Input: part model. Units: mm. Frame: model coordinates. A direction names the side the tool comes from. Give positions to 0.01 mm unless a question says otherwise; leave off trailing zeros. Write each loop counter-clockwise with the first axis right and the second up, starting at its lowest first coordinate (ties: lowest second). Pieces come first, ordered by that corner, then holes. Notation, with made-up numbers: (-38.75, 70) - (17.25, 70) arc R33 ccw to (17.25, 106) - close; hole circle Ø10 at (3, 30.25). An arc over 180 degrees is marked (long way). Use a Markdown table: item, result. Add a question column.
1. Material intervals for probe 1 along X at (y, z) = (3.6, -5); probe 2 along X at (y, z) = (1.4, 25.5); probe 3 along Z at (x, y) = (6, 1.45), sorted ascending.
2. Section query A-A, the plane z = 6.5. Return loops of the section in (x, y).
3. Mould query, pull axis X, two halves, no side actions, for faces 1 (the flat face through (13.804, 1.972, 24.362)), 2 (the flat face through (-28, 2, 0)), 3 (the flat face through (-13, 4, 24)), 4 (the flat face through (-13.21, 1.97, -23.32)). Classes: released by +X, released by -X, zero draft, split by the parting line, or undercut.
4. Set-up query: faces 5 (the flat face through (26.8, 2, 0)), 6 (the flat face through (-13.804, 1.972, -24.362)). Return all of +Z, -Z, +X, -X, +Y, -Y with unobstructed straight access to the full face (end or side cutting, diameter ignored); none if empty.
5. Section query B-B, the plane x = -2.5. Return loops of the section in (y, z), plus the area to 3 significant figures.
6. Pin query (flat end, axial travel): pin 1 (1.5 mm diameter, centred on x = 17.5, y = 2.5, fed in from +Z). Return the tip coordinate at first contact, or that it passes through.
```python
from build123d import *

# Parameters (mm, degrees)
RESSALTO_EXTRUS_O1_DEPTH = 4
ESBO_O2_R                = 1
CORTE_EXTRUS_O1_DEPTH    = 71.578561429


with BuildPart() as part:
    # Esboço1 → Ressalto-extrusão1 (new body)
    with BuildSketch(Plane(origin=(0, 0, 0), x_dir=(1, 0, 0), z_dir=(0, 1, 0))):
        Polygon((28, -16.165807537), (28, 16.165807537), (0, 32.331615075), (-28, 16.165807537), (-28, -16.165807537), (0, -32.331615075), align=None)
        Polygon((26.8, 15.472987214), (0, 30.945974429), (-26.8, 15.472987214), (-26.8, -15.472987214), (0, -30.945974429), (26.8, -15.472987214), align=None, mode=Mode.SUBTRACT)
    extrude(amount=RESSALTO_EXTRUS_O1_DEPTH)

    # Esboço2 → Corte-extrusão1 (cut, through all)
    with BuildSketch(Plane(origin=(-14, 0, 24.248711306), x_dir=(0.8660254037844387, 0, 0.49999999999999994), z_dir=(-0.4999999999999999, 0, 0.8660254037844386))):
        with Locations((0, 2)):
            Circle(ESBO_O2_R)
    extrude(amount=-CORTE_EXTRUS_O1_DEPTH, mode=Mode.SUBTRACT)


solid = part.part
```
Result sheet:
| question | item | result |
|---|---|---|
| 1 | probe 1 | x = -28 to -26.8, 26.8 to 28 |
| 1 | probe 2 | x = -11.83 to -9.43, 9.43 to 11.83 |
| 1 | probe 3 | z = -28.87 to -27.48, 27.48 to 28.87 |
| 2 | outline | (-28, 0) - (-26.8, 0) - (-26.8, 4) - (-28, 4) - close; (26.8, 0) - (28, 0) - (28, 4) - (26.8, 4) - close |
| 3 | face 1 | released by +X |
| 3 | face 2 | released by -X |
| 3 | face 3 | zero draft |
| 3 | face 4 | undercut |
| 4 | face 5 | +Y, -Y |
| 4 | face 6 | -Z, -X, +Y, -Y |
| 5 | outline | (0, -30.89) - (4, -30.89) - (4, -29.5) - (0, -29.5) - close; (0, 29.5) - (4, 29.5) - (4, 30.89) - (0, 30.89) - close |
| 5 | area | 11.1 mm² |
| 6 | pin 1 | stops at z = 22.66 |
